Build history of the part. All positions in model axes, mm. A direction names the side the tool comes from. Round coordinates to 2 decimals unless told otherwise and drop trailing zeros. Write each loop counter-clockwise with the first axis right and the second up, starting at its lowest first coordinate (ties: lowest second). Pieces come first, ordered by that corner, then holes. Notation, with made-up numbers: (80, 27) -> (134, 27) arc R11 cw to (134, 47) -> close; hole circle Ø7 at (38.5, 2.25). An arc over 180 degrees is marked (long way). Answer in a Markdown table with one row per item. Add a question column.
from build123d import *

# Parameters (mm, degrees)
F0_R     = 15
F1_DEPTH = 75
F2_R     = 5
F3_DEPTH = 15
F4_R     = 10
F5_DEPTH = 25


with BuildPart() as f1:
    # F0 (on Top) → F1 (new body)
    with BuildSketch(Plane.XY):
        with BuildLine():
            Line((-50, -25), (0, -25))
            ThreePointArc((0, -25), (17.67767, -17.67767), (25, 0))
            Line((25, 0), (25, 10))
            Line((25, 10), (70, 10))
            Line((70, 10), (70, 25))
            Line((70, 25), (0, 25))
            ThreePointArc((0, 25), (-17.67767, 17.67767), (-25, 0))
            Line((-25, 0), (-25, -15))
            Line((-25, -15), (-40, -15))
            Line((-40, -15), (-40, 50.105155))
            Line((-40, 50.105155), (-50, 50.105155))
            Line((-50, 50.105155), (-50, -25))
        make_face()
        Circle(F0_R, mode=Mode.SUBTRACT)
    extrude(amount=F1_DEPTH)

    # F2 (on face) → F3 (cut)
    with BuildSketch(Plane(origin=(0, 25, 0), x_dir=(-1, 0, 0), z_dir=(0, 1, 0))):
        with Locations((-55, 20)):
            Circle(F2_R)
        with Locations((-55, 55)):
            Circle(F2_R)
    extrude(amount=-F3_DEPTH, mode=Mode.SUBTRACT)

    # F4 (on face) → F5 (cut)
    with BuildSketch(Plane.YZ.offset(-40)):
        with Locations((15.194554, 40)):
            Circle(F4_R)
        Polygon((35.105155, 75), (50.105155, 60), (50.105155, 75), align=None)
        Polygon((50.105155, 0), (50.105155, 15), (35.105155, 0), align=None)
    extrude(amount=-F5_DEPTH, mode=Mode.SUBTRACT)


solid = f1.part
(1) Saw through at C-C (x = -9.5). List the corners of the cut face in (y, z), plus the area to 3 significant figures.
(2) Saw through at D-D (z = 70.5). List the corners of the cut face in (x, y).
(3) Which spindle directions (+Z, -Z, +X, -X, +Y, -Y) get a long thin tool onto all of the face, cutting with end or side? Do faces 4 (the face through (35, 25, 37)), 5 (the face through (25, 5, 37)), 6 (the face through (-32, -15, 37)). Say none if no direction does.
(4) Saw through at B-B (x = 55). List the corners of the cut face in (y, z).
(5) Drop flat-ended pins along their axis: P1, Ø16, axis at x = 55, z = 20, coming from the +Y side; P2, Ø16, axis at x = 55, z = 55, coming from the -Y side; P3, Ø5, axis at y = 6, z = 24, coming from the +X side. Give the stop position or say it passes through.
(6) Mould opens along Z. For faces 1 (the face through (-18, 5, 75)), 2 (the face through (70, 17, 37)), 3 (the face through (-44.93, 13.027, 30.238)) say: pulls with the +Z half, pulls with the -Z half, needs draft (parallel to the pull), parting line crosses it, or undercut.
(7) Probe line 1 along Z through (x, y) = (55, 15); line 2 along X through (y, z) = (-11.5, 45); line 3 along X through (y, z) = (5.5, 63). List the from-to ranges inside material, lowest first.
(8) Saw through at A-A (z = 55). List the corners of the cut face in (x, y), plus the area to 3 significant figures.
Answer sheet:
| question | item | result |
|---|---|---|
| 1 | outline | (-25, 0) -> (-11.61, 0) -> (-11.61, 75) -> (-25, 75) -> close; (11.61, 0) -> (23.12, 0) -> (23.12, 75) -> (11.61, 75) -> close |
| 1 | area | 1,870 mm² |
| 2 | outline | (-50, -25) -> (0, -25) arc R25 ccw to (25, 0) -> (25, 10) -> (70, 10) -> (70, 25) -> (0, 25) arc R25 ccw to (-25, 0) -> (-25, -15) -> (-40, -15) -> (-40, 39.61) -> (-50, 39.61) -> close; hole circle Ø30 at (0, 0) |
| 3 | face 4 | +Z, -Z, +X, +Y |
| 3 | face 5 | +Z, -Z, +X, -Y |
| 3 | face 6 | +Z, -Z, +Y |
| 4 | outline | (10, 0) -> (25, 0) -> (25, 15) -> (10, 15) -> close; (10, 25) -> (25, 25) -> (25, 50) -> (10, 50) -> close; (10, 60) -> (25, 60) -> (25, 75) -> (10, 75) -> close |
| 5 | P1 | stops at y = 25 |
| 5 | P2 | stops at y = 10 |
| 5 | P3 | stops at x = 25 |
| 6 | face 1 | pulls with the +Z half |
| 6 | face 2 | needs draft |
| 6 | face 3 | undercut |
| 7 | line 1 | z = 0 to 15, 25 to 50, 60 to 75 |
| 7 | line 2 | x = -50 to -40, -25 to -9.63, 9.63 to 22.2 |
| 7 | line 3 | x = -50 to -40, -24.39 to -13.96, 13.96 to 25 |
| 8 | outline | (-50, -25) -> (0, -25) arc R25 ccw to (25, 0) -> (25, 10) -> (50, 10) -> (50, 25) -> (0, 25) arc R25 ccw to (-25, 0) -> (-25, -15) -> (-40, -15) -> (-40, 50.11) -> (-50, 50.11) -> close; (60, 10) -> (70, 10) -> (70, 25) -> (60, 25) -> close; hole circle Ø30 at (0, 0) |
| 8 | area | 2,950 mm² |
